Build history of the part. All positions in model axes, mm. A direction names the side the tool comes from. Coordinates: 2 decimals unless noted, no trailing zeros. Order: outer loops, then holes, each group sorted by start corner. A loop starts at its lowest first (then second) coordinate and runs counter-clockwise, first axis right, second up. Notation, with made-up numbers: M 35,38.25 L 60,38.25 A28 cw 60,65.25 Z; hole C 70.5,35.5 d3. An arc over 180 degrees is marked long. Write item = value, one per line. Start each with the question number.
Q1. Band-saw the part on B-B on x = -282. Write the cut outline in (y, z).
Q2. Band-saw the part on D-D on z = -35. Write the cut outline in (x, y).
Q3. Pull direction X, two halves, no side cores. Call faces 3 (the face through (-381, -2, -150)), 4 (the face through (381, -2, -150)), 5 (the face through (-288, 1, -279.4)), 6 (the face through (-5, 2, -304.8)): released by +X, released by -X, zero draft, split by the parting line, or undercut.
Q4. 3-axis set-ups, long thin cutter, end or side, ignore diameter. For faces 1 (the face through (-5, -152.4, -150)), 2 (the face through (-157, 41, -76.2)): which of +Z, -Z, +X, -X, +Y, -Y reach the whole face in a straight line?
Q5. Pin check, flat tip, straight feed: P1, Ø15.5, axis at x = -149.5, y = -51, coming from the +Z side. Stop position of the tip, or through.
Q6. Band-saw the part on A-A on z = -100. Write the cut outline in (x, y), plus the area to 3 significant figures.
Q7. Band-saw the part on C-C on y = -97. Write the cut outline in (x, z), plus the area to 3 significant figures.
Q8. Drill centre lines: probe 1 along X at (y, z) = (-43.5, -142); probe 2 along Y at (x, z) = (-223, -260); probe 3 along Z at (x, y) = (-209.5, -28). Where is each one in solid material? Low to high.
```python
from build123d import *

# Parameters (mm, degrees)
F0_W     = 762
F0_H     = 304.8
F1_DEPTH = 304.8
F2_W     = 163.013741
F2_H     = 278.260633
F3_DEPTH = 279.4
F4_R     = 26.093017
F4_R_2   = 25.87402
F5_DEPTH = 76.2


with BuildPart() as f1:
    # F0 (on Top) → F1 (new body)
    with BuildSketch(Plane.XY):
        Rectangle(F0_W, F0_H)
    extrude(amount=-F1_DEPTH)

    # F2 (on face) → F3 (cut)
    with BuildSketch(Plane.XY):
        with Locations((-287.166662, -0.719539)):
            Rectangle(F2_W, F2_H)
    extrude(amount=-F3_DEPTH, mode=Mode.SUBTRACT)

    # F4 (on face) → F5 (cut)
    with BuildSketch(Plane.XY):
        with Locations((-156.819597, 40.271699)):
            Circle(F4_R)
        with Locations((-156.819597, -56.807101)):
            Circle(F4_R_2)
    extrude(amount=-F5_DEPTH, mode=Mode.SUBTRACT)


solid = f1.part
```
Recorded:
q1.outline = M -152.4,-304.8 L 152.4,-304.8 L 152.4,0 L 138.41,0 L 138.41,-279.4 L -139.85,-279.4 L -139.85,0 L -152.4,0 Z
q2.outline = M -381,-152.4 L 381,-152.4 L 381,152.4 L -381,152.4 Z; hole M -368.67,-139.85 L -205.66,-139.85 L -205.66,138.41 L -368.67,138.41 Z; hole C -156.82,40.27 d52.19; hole C -156.82,-56.81 d51.75
q3.face_3 = released by -X
q3.face_4 = released by +X
q3.face_5 = undercut
q3.face_6 = zero draft
q4.face_1 = +Z, -Z, +X, -X, -Y
q4.face_2 = +Z
q5.P1 = -76.2
q6.outline = M -381,-152.4 L 381,-152.4 L 381,152.4 L -381,152.4 Z; hole M -368.67,-139.85 L -205.66,-139.85 L -205.66,138.41 L -368.67,138.41 Z
q6.area = 187,000 mm2
q7.outline = M -381,-304.8 L 381,-304.8 L 381,0 L -205.66,0 L -205.66,-279.4 L -368.67,-279.4 L -368.67,0 L -381,0 Z
q7.area = 187,000 mm2
q8.probe_1 = -381 to -368.67, -205.66 to 381
q8.probe_2 = -152.4 to -139.85, 138.41 to 152.4
q8.probe_3 = -304.8 to -279.4
